Check sheet for the drawn part. Datum: minimum x, y, z corner. Units: mm. Round coordinates to 2 decimals unless told otherwise and drop trailing zeros. Write each loop counter-clockwise with the first axis right and the second up, starting at its lowest first coordinate (ties: lowest second). Pieces come first, ordered by that corner, then holes. Notation, with made-up numbers: (43, -22.75) - (52, -22.75) arc R16 ccw to (52, -7.75) - close; hole circle Ø7 at (86.5, 33.5). An arc over 180 degrees is marked (long way). Answer as a JSON object with one key per item and string values.
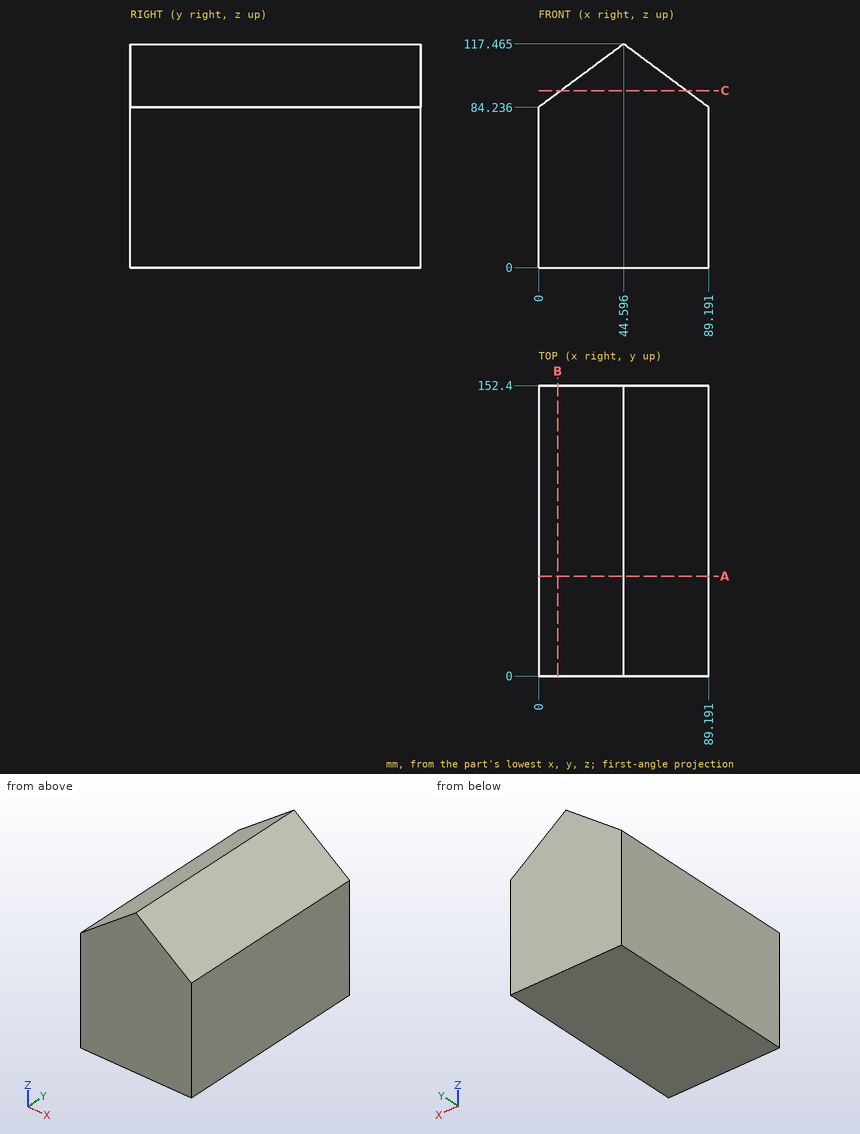
Q1. Section check B-B, the plane x = 10. Record the cut outline in (y, z).
Geometry check:
{"outline": "(0, 0) - (152.4, 0) - (152.4, 91.69) - (0, 91.69) - close"}
Q2. Gauge pin test, flat ends, axial feed: P1, Ø5, axis at y = 124, z = 89, coming from the -X side; P2, Ø10, axis at y = 59.5, z = 105, coming from the +X side (1 decimal); P3, Ø3, axis at y = 77.5, z = 103.5, coming from the +X side. Record the tip position at first contact, or that the pin passes through.
Geometry check:
{"P1": "stops at x = 3.04", "P2": "stops at x = 68", "P3": "stops at x = 65.35"}
Q3. Section check A-A, the plane y = 52.5. Record the cut outline in (x, z) (1 decimal).
Geometry check:
{"outline": "(0, 0) - (89.2, 0) - (89.2, 84.2) - (44.6, 117.5) - (0, 84.2) - close"}
Q4. Section check C-C, the plane z = 93. Record the cut outline in (x, y), then the cut area to 3 significant figures.
Geometry check:
{"outline": "(11.76, 0) - (77.43, 0) - (77.43, 152.4) - (11.76, 152.4) - close", "area": "10,000 mm2"}
Q5. Material ranges on line 1 along Z through (x, y) = (13.5, 23) (1 decimal); line 2 along Z through (x, y) = (53.5, 117.5), recorded low to high. Write a range as [from, to].
Geometry check:
{"line 1": "z = [0, 94.3]", "line 2": "z = [0, 110.83]"}
